Autodesk Inventor part; units mm, degrees
ref_plane "YZ Plane" through (0, 0, 0) normal (1, 0, 0) x (0, 1, 0)
ref_plane "XZ Plane" through (0, 0, 0) normal (0, 1, 0) x (-1, 0, 0)
ref_plane "XY Plane" through (0, 0, 0) normal (0, 0, 1) x (1, 0, 0)
sketch "Sketch1" plane through (0, 0, 0) normal (0, 0, 1) x (1, 0, 0)
  line L0 (-30, 30) -> (30, 30)
  line L1 (30, 30) -> (30, -30)
  line L2 (30, -30) -> (-30, -30)
  line L3 (-30, -30) -> (-30, 30)
  line L4 (-30, 30) -> (30, -30) construction
  line L5 (30, 30) -> (-30, -30) construction
  circle A0 centre (-24, 24) radius 1.65
  circle A1 centre (-24, -24) radius 1.65
  circle A2 centre (24, -24) radius 1.65
  circle A3 centre (24, 24) radius 1.65
  point P0 (0, 0)
  dimension "d0" = 60
  dimension "d1" = 60
  dimension "d2" = 3.3
  dimension "d3" = 24
  dimension "d6" = 360
extrude "Extrusion1" add sketch "Sketch1" along normal blind 4
properties part number "antenna_socket_cap" material "Acetal Resin, Black"
Input: part model. Units: mm. Frame: model coordinates. Round coordinates to 2 decimals unless told otherwise and drop trailing zeros. Loops run counter-clockwise (first coordinate to the right, second up) from the corner with the lowest first, then second, coordinate; pieces in that order, holes last. Notation, with made-up numbers: M -23,46 L 17,46 A28 ccw 17,68 Z; hole C -5,62.25 d1. An arc over 180 degrees is marked long. Answer in a Markdown table with one row per item. Add a question column.
1. Section A-A (y = -24). Output: boundary loops of the cut face in (x, z), and give its area (3 significant figures).
2. Ray query, probe 1 along Y at (x, z) = (-24, 0.9); probe 2 along X at (y, z) = (23.5, 2.65). Return the intervals inside material, ascending.
3. Contact query for a flat-ended pin moving along its axis: pin 1 (2 mm diameter, centred on x = -24, y = -24, fed in from +Z). Output: stop coordinate, or through.
4. Mould query, pull axis X, two halves, no side actions, for faces 1 (the face through (22.784, -25.115, 1.972)), 2 (the face through (-30, 0, 2)), 3 (the face through (-25.216, -25.115, 1.972)), 4 (the face through (0, 0, 0)). Classes: released by +X, released by -X, zero draft, split by the parting line, or undercut.
Values follow:
| question | item | result |
|---|---|---|
| 1 | outline | M -30,0 L -25.65,0 L -25.65,4 L -30,4 Z; M -22.35,0 L 22.35,0 L 22.35,4 L -22.35,4 Z; M 25.65,0 L 30,0 L 30,4 L 25.65,4 Z |
| 1 | area | 214 mm^2 |
| 2 | probe 1 | -30 to -25.65, -22.35 to 22.35, 25.65 to 30 |
| 2 | probe 2 | -30 to -25.57, -22.43 to 22.43, 25.57 to 30 |
| 3 | pin 1 | through |
| 4 | face 1 | undercut |
| 4 | face 2 | released by -X |
| 4 | face 3 | undercut |
| 4 | face 4 | zero draft |
